from build123d import *

# Parameters (mm, degrees)
BOSS_EXTRUDE1_DEPTH      = 14
SKETCH2_R                = 1
BOSS_EXTRUDE2_DEPTH      = 9
BOSS_EXTRUDE3_DEPTH      = 6
BOSS_EXTRUDE3_DEPTH_BACK = 6
SKETCH3_W                = 1
SKETCH3_H                = 10
SKETCH4_R                = 2
SKETCH4_R_2              = 1.5
BOSS_EXTRUDE4_DEPTH      = 0.75
SKETCH5_R                = 1.5
BOSS_EXTRUDE5_DEPTH      = 3.5
BOSS_EXTRUDE6_DEPTH      = 6
BOSS_EXTRUDE7_DEPTH      = 1
FILLET1_R                = 1
FILLET2_R                = 0.75


with BuildPart() as part:
    # Sketch1 → Boss-Extrude1 (new body)
    with BuildSketch(Plane.XY):
        with BuildLine():
            Line((3.25, 4.74341649), (-3.25, 4.74341649))
            ThreePointArc((-3.25, 4.74341649), (-5.086747487, 2.680951324), (-5.75, 0))
            Line((-5.75, 0), (5.75, 0))
            ThreePointArc((5.75, 0), (5.086747487, 2.680951324), (3.25, 4.74341649))
        make_face()
        with BuildLine():
            Line((5.75, 0), (-5.75, 0))
            ThreePointArc((-5.75, 0), (-5.086747487, -2.680951324), (-3.25, -4.74341649))
            Line((-3.25, -4.74341649), (3.25, -4.74341649))
            ThreePointArc((3.25, -4.74341649), (5.086747487, -2.680951324), (5.75, 0))
        make_face()
    extrude(amount=BOSS_EXTRUDE1_DEPTH)

    # Sketch2 → Boss-Extrude2 (add)
    with BuildSketch(Plane.XY):
        with Locations((4, -3.24341649)):
            Circle(SKETCH2_R)
        with Locations((-4, 3.24341649)):
            Circle(SKETCH2_R)
    extrude(amount=-BOSS_EXTRUDE2_DEPTH)

    # Sketch3 → Boss-Extrude3 (add, two sides: drawn at the far end of the back side and taken through both)
    with BuildSketch(Plane(origin=(0, 0, 0), x_dir=(0, 0, -1), z_dir=(1, 0, 0)).offset(-BOSS_EXTRUDE3_DEPTH_BACK)):
        with Locations((0.5, 0)):
            Rectangle(SKETCH3_W, SKETCH3_H)
        with Locations((4.459742397, 0)):
            Rectangle(SKETCH3_W, SKETCH3_H)
        with Locations((8.5, 0)):
            Rectangle(SKETCH3_W, SKETCH3_H)
    extrude(amount=BOSS_EXTRUDE3_DEPTH + BOSS_EXTRUDE3_DEPTH_BACK)

    # Sketch4 → Boss-Extrude4 (add)
    with BuildSketch(Plane(origin=(0, 0, -9), x_dir=(-1, 0, 0), z_dir=(0, 0, -1))):
        with Locations(Location((0, 0, 0), (0, 0, 180))):
            Circle(SKETCH4_R)
        Circle(SKETCH4_R_2, mode=Mode.SUBTRACT)
    extrude(amount=BOSS_EXTRUDE4_DEPTH)

    # Sketch5 → Boss-Extrude5 (add)
    with BuildSketch(Plane(origin=(0, 0, -9), x_dir=(-1, 0, 0), z_dir=(0, 0, -1))):
        Circle(SKETCH5_R)
    extrude(amount=BOSS_EXTRUDE5_DEPTH)

    # Sketch6 → Boss-Extrude6 (add)
    with BuildSketch(Plane(origin=(0, 0, -12.5), x_dir=(-1, 0, 0), z_dir=(0, 0, -1))):
        with BuildLine():
            Line((1.25, 0.829156198), (-1.25, 0.829156198))
            ThreePointArc((-1.25, 0.829156198), (-0.433012702, -1.436140662), (1.5, 0))
            ThreePointArc((1.5, 0), (1.436140662, 0.433012702), (1.25, 0.829156198))
        make_face()
    extrude(amount=BOSS_EXTRUDE6_DEPTH)

    # Sketch7 → Boss-Extrude7 (add)
    with BuildSketch(Plane.XY.offset(14)):
        with BuildLine():
            Line((-3.187454564, -4.54341649), (3.187454564, -4.54341649))
            ThreePointArc((3.187454564, -4.54341649), (5.55, 0), (3.187454564, 4.54341649))
            Line((3.187454564, 4.54341649), (-3.187454564, 4.54341649))
            ThreePointArc((-3.187454564, 4.54341649), (-5.55, 0), (-3.187454564, -4.54341649))
        make_face()
    extrude(amount=BOSS_EXTRUDE7_DEPTH)

    # Fillet1
    fillet1_edges = [part.edges().sort_by_distance(p)[0] for p in [
        (0, 4.54341649, 15),
        (5.55, 0, 15),
        (0, -4.54341649, 15),
        (-5.55, 0, 15),
    ]]
    fillet(fillet1_edges, radius=FILLET1_R - 0.0001)  # a hair under: the kernel refuses the full size

    # Fillet2
    fillet2_edges = [part.edges().sort_by_distance(p)[0] for p in [
        (-6, 5, -0.5),
        (-6, -5, -0.5),
        (6, -5, -0.5),
        (6, 5, -0.5),
        (-6, 5, -4.459742397),
        (-6, -5, -4.459742397),
        (6, -5, -4.459742397),
        (6, 5, -4.459742397),
        (-6, -5, -8.5),
        (-6, 5, -8.5),
        (6, 5, -8.5),
        (6, -5, -8.5),
    ]]
    fillet(fillet2_edges, radius=FILLET2_R)


solid = part.part
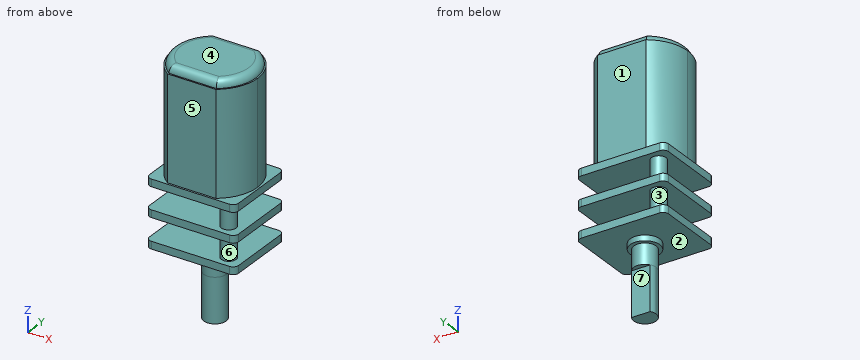
The model under review builds one solid part; all positions refer to its coordinate system, in mm. Face numbers are marked on the shaded views. A direction names the side the tool comes from. Give positions to 0.01 mm unless a question says otherwise; leave off trailing zeros. Write each loop counter-clockwise with the first axis right and the second up, starting at its lowest first coordinate (ties: lowest second). Pieces come first, ordered by that corner, then holes. Notation, with made-up numbers: M 14,29.25 L 72,29.25 A15 ccw 72,52.25 Z; hole C -37,72.5 d2. An arc over 180 degrees is marked long. One line per question, with ' | ' between items. Start each with the question number.
Item 1: Wall thickness on line 1 (Z direction, x = 5.25, y = 2.75); line 2 (Z direction, x = -2.5, y = -2.5); line 3 (Y direction, x = -1.25, z = 10.5): over which ranges is each line inside the solid? List them lowest first. Write a range as from..to.
Item 2: We need section B-B on z = 0.5. Write out the cut boundary in (x, y), plus the area to 3 significant figures.
Item 3: We need section A-A on x = 0. Give the number of separate pieces and of enclosed holes in the cut face, plus the area to 3 significant figures.
Item 4: For pin 1 (3.5 mm diameter, centred on x = -1.5, z = 7.5, fed in from +Y); pin 2 (5 mm diameter, centred on x = -1, y = 2.5, fed in from -Z); pin 3 (2 mm diameter, centred on x = -1, z = 6, fed in from -Y); pin 4 (0.5 mm diameter, centred on x = 0.5, y = 1.5, fed in from -Z), all flat-tipped, find the tip position at first contact; note any pin that passes through.
Item 5: For the marked faces 5, 6 and 7, list the 3-axis set-ups (+Z, -Z, +X, -X, +Y, -Y) from which the entire face can be reached by the end or side of a thin tool; tool diameter is ignored.
Item 6: Draft analysis for pull direction Z (two halves, no side actions). For the marked faces 1, 2, 3 and 4, state which applies: released by +Z, released by -Z, zero draft, split by the parting line, or undercut.
Results found:
1) line 1: z = -9..-8, -4.96..-3.96, -1..0 | line 2: z = -9..-8, -4.96..-3.96, -1..15 | line 3: y = -4.74..4.74
2) outline: M -3.25,-4.74 L 3.25,-4.74 A5.75 ccw 3.25,4.74 L -3.25,4.74 A5.75 ccw Z | area: 95.0 mm2
3) separate pieces: 3 | enclosed holes: 0 | area: 197 mm2
4) pin 1: stops at y = 4.74 | pin 2: stops at z = -18.5 | pin 3: stops at y = -4.74 | pin 4: stops at z = -12.5
5) face 5: +Z, +X, -X, -Y | face 6: none | face 7: -Z, +X, -X, +Y
6) face 1: zero draft | face 2: released by -Z | face 3: undercut | face 4: released by +Z
